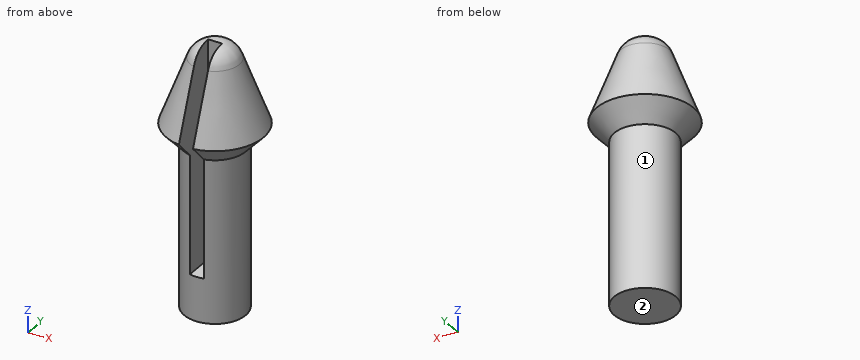
```python
from build123d import *

# Parameters (mm, degrees)
F4_R      = 1.905
F2_R      = 3.81
F5_FACE_R = 3.81
F0_R      = 2.40665
F7_DEPTH  = 12.7
F12_W     = 1.1028264416
F12_H     = 38.8027336448
F13_DEPTH = 25.4


with BuildPart() as f5:
    # F4 (on offset) → F5 section 0
    with BuildSketch(Plane.XY.offset(6.604)):
        Circle(F4_R)
    # F2 (on offset) → F5 section 1
    with BuildSketch(Plane.XY.offset(1.524)):
        Circle(F2_R)
    loft()

    # F5_face (on face) → F6 section 0
    with BuildSketch(Plane(origin=(0, 0, 1.524), x_dir=(1, 0, 0), z_dir=(0, 0, -1))):
        Circle(F5_FACE_R)
    # F0 (on Top) → F6 section 1
    with BuildSketch(Plane.XY):
        Circle(F0_R)
    loft()

    # F0 (on Top) → F7 (join)
    with BuildSketch(Plane.XY):
        Circle(F0_R)
    extrude(amount=-F7_DEPTH)

    # F9 (on Front) → F11 (revolve)
    with BuildSketch(Plane.XZ):
        with BuildLine():
            Line((0, 6.604), (0, 7.8187098284))
            ThreePointArc((0, 7.8187098284), (-1.1744726921, 7.5594693104), (-1.905, 6.604))
            Line((-1.905, 6.604), (0, 6.604))
        make_face()
    revolve(axis=Axis((0, 0, 7.2099673588), (0, 0, -1)))

    # F12 (on Front) → F13 (cut)
    with BuildSketch(Plane.XZ):
        with Locations((0, 10.1560307667)):
            Rectangle(F12_W, F12_H)
    extrude(amount=F13_DEPTH, mode=Mode.SUBTRACT)


solid = f5.part
```
CAD build for the part. Positions are in the model's coordinates, mm. Face numbers are marked on the shaded views. A direction names the side the tool comes from. Coordinates: 2 decimals unless noted, no trailing zeros. Order: outer loops, then holes, each group sorted by start corner. A loop starts at its lowest first (then second) coordinate and runs counter-clockwise, first axis right, second up. Notation, with made-up numbers: M 7,36.25 L 36,36.25 A8 cw 36,51.25 Z; hole C 66.25,47 d2. An arc over 180 degrees is marked long. Write each question's results on one line, items separated by ' | '. Start each with the question number.
Q1. Cut at C-C (z = -7.25). List the corners of the cut face in (x, y).
Q2. Cut at A-A (z = -10.75). List the corners of the cut face in (x, y).
Q3. Flat gauge pins, fed straight in: P1, Ø1.2, axis at x = 0, z = -4, coming from the -Y side; P2, Ø0.6, axis at x = 0, y = -1, coming from the +Z side; P3, Ø2, axis at x = 1, z = 5.5, coming from the +Y side. Where does each tip first touch, or does it go through?
Q4. Drill centre lines: probe 1 along X at (y, z) = (-0.5, -4.75); probe 2 along X at (y, z) = (-1.25, -0.75); probe 3 along Z at (x, y) = (-1.75, -1.75). Where is each one in solid material? Low to high. Write a range as from..to.
Q5. Which spindle directions (+Z, -Z, +X, -X, +Y, -Y) get a long thin tool onto all of the face, cutting with end or side? Do the marked faces 1 and 2. Say none if no direction does.
Q6. Cut at B-B (z = 0.75). List the corners of the cut face in (x, y).
Found:
1) outline: M -0.55,-2.34 L -0.55,0 L 0.55,0 L 0.55,-2.34 A2.41 ccw long Z
2) outline: C 0,0 d4.81
3) P1: y = -2.34 | P2: z = -9.25 | P3: y = 2.6
4) probe 1: -2.35..-0.55, 0.55..2.35 | probe 2: -2.06..-0.55, 0.55..2.06 | probe 3: 0.07..5.08
5) face 1: -Z | face 2: -Z, +X, -X, +Y, -Y
6) outline: M -0.55,-3.05 L -0.55,0 L 0.55,0 L 0.55,-3.05 A3.1 ccw long Z
